```python
from build123d import *

# Parameters (mm, degrees)
F0_W           = 6
F0_H           = 3
F1_DEPTH       = 16
F3_D           = 2
F3_DEPTH       = 5
F3_CBORE_D     = 4
F3_CBORE_DEPTH = 1
F3_TIP         = 0.600860619
F5_D           = 2
F5_DEPTH       = 5
F5_CBORE_D     = 4
F5_CBORE_DEPTH = 1
F5_TIP         = 0.600860619
F6_SIZE        = 4
F8_D           = 3
F8_CBORE_D     = 6
F8_CBORE_DEPTH = 1
F9_SIZE        = 1
F10_SIZE       = 2


with BuildPart() as f1:
    # F0 (on Front) → F1 (new body, symmetric)
    with BuildSketch(Plane.XZ):
        with Locations((-6, 17.5)):
            Rectangle(F0_W, F0_H)
        Polygon((0, -19), (0, 19), (-3, 19), (-3, 16), (-3, -16), (-3, -19), align=None)
        with Locations((-6, -17.5)):
            Rectangle(F0_W, F0_H)
    extrude(amount=F1_DEPTH, both=True)

    # F3
    with Locations(Plane.XY.offset(19)):
        with Locations((-5.5, 8), (-5.5, -8)):
            CounterBoreHole(F3_D / 2, F3_CBORE_D / 2, F3_CBORE_DEPTH, depth=F3_DEPTH)
            with Locations((0, 0, -(F3_DEPTH + F3_TIP / 2))):  # 118° drill point
                Cone(0, F3_D / 2, F3_TIP, mode=Mode.SUBTRACT)

    # F5
    with Locations(Plane(origin=(0, 0, -19), x_dir=(1, 0, 0), z_dir=(0, 0, -1))):
        with Locations((-5.5, -8), (-5.5, 8)):
            CounterBoreHole(F5_D / 2, F5_CBORE_D / 2, F5_CBORE_DEPTH, depth=F5_DEPTH)
            with Locations((0, 0, -(F5_DEPTH + F5_TIP / 2))):  # 118° drill point
                Cone(0, F5_D / 2, F5_TIP, mode=Mode.SUBTRACT)

    # F6
    f6_edges = [f1.edges().sort_by_distance(p)[0] for p in [
        (-9, -16, 17.5),
        (-9, 16, 17.5),
        (-9, 16, -17.5),
        (-9, -16, -17.5),
    ]]
    chamfer(f6_edges, length=F6_SIZE)

    # F8 (through all)
    with Locations(Plane(origin=(-3, 0, 0), x_dir=(0, -1, 0), z_dir=(-1, 0, 0))):
        with Locations((0, 8), (0, -8)):
            CounterBoreHole(F8_D / 2, F8_CBORE_D / 2, F8_CBORE_DEPTH)

    # F9
    f9_edges = [f1.edges().sort_by_distance(p)[0] for p in [
        (-2.5, 16, 19),
        (-7, 14, 19),
        (-9, 0, 19),
        (-7, -14, 19),
        (-2.5, -16, 19),
        (-2.5, 16, -19),
        (-7, 14, -19),
        (-9, 0, -19),
        (-7, -14, -19),
        (-2.5, -16, -19),
    ]]
    chamfer(f9_edges, length=F9_SIZE)

    # F10
    f10_edges = [f1.edges().sort_by_distance(p)[0] for p in [
        (0, 16, 0),
        (0, -16, 0),
    ]]
    chamfer(f10_edges, length=F10_SIZE)


solid = f1.part
```
The model under review builds one solid part; all positions refer to its coordinate system, in mm. A direction names the side the tool comes from. Give positions to 0.01 mm unless a question says otherwise; leave off trailing zeros. Write each loop counter-clockwise with the first axis right and the second up, starting at its lowest first coordinate (ties: lowest second). Pieces come first, ordered by that corner, then holes. Notation, with made-up numbers: (4.25, 27) - (46.25, 27) arc R35 cw to (46.25, 66) - close; hole circle Ø6 at (42, 22). An arc over 180 degrees is marked (long way). Answer in a Markdown table with one row per item. Add a question column.
1. We need section C-C on y = -4.5. Write out the cut boundary in (x, z).
2. We need section A-A on z = -8. Write out the cut boundary in (x, y), then the cut area to 3 significant figures.
3. Insertion check: P1, Ø3, axis at x = -5.5, y = 8, coming from the +Z side; P2, Ø1.5, axis at y = 12.5, z = 8.5, coming from the -X side; P3, Ø1.2, axis at x = -5, y = -8.5, coming from the -Z side; P4, Ø1.6, axis at x = -5.5, y = 8, coming from the -Z side. Each pin has a flat end and moves straight along its axis. Give the tip position at first contact, or say it passes through.
4. We need section D-D on z = -14. Write out the cut boundary in (x, y).
5. Tool access review of faces 5 (the flat face through (-4.6, 7.1, 18)), 6 (the flat face through (-3, -15.5, -18.5)), 7 (the flat face through (-7, -14, 17)), 8 (the flat face through (-6, 0, 16)), 9 (the flat face through (-4.6, -7.1, -18)): name each direction out of +Z, -Z, +X, -X, +Y, -Y from which nothing blocks a thin tool from reaching the whole face with its end or side.
6. We need section B-B on y = 8. Write out the cut boundary in (x, z), then the cut area to 3 significant figures.
7. Draft analysis for pull direction X (two halves, no side actions). For faces 1 (the flat face through (0, 0, 0)), 2 (the flat face through (-3, 15.5, 18.5)), 3 (the cylindrical face through (-5.37, 8.99, 16.99)), 4 (the cylindrical face through (-5.37, 7.01, -16.99)), state which applies: +X half, -X half, draft (parallel to the pull), parting line (faces both ways), or undercut.
8. Wall thickness on line 1 along Z through (x, y) = (-2.6, 0); line 2 along Z through (x, y) = (-5.5, 5.5); line 3 along Z through (x, y) = (-0.45, 0): over which ranges is each line inside the solid? List them lowest first. Write a range as [from, to].
Ans:
| question | item | result |
|---|---|---|
| 1 | outline | (-9, -18) - (-8, -19) - (0, -19) - (0, 19) - (-8, 19) - (-9, 18) - (-9, 16) - (-3, 16) - (-3, -16) - (-9, -16) - close |
| 2 | outline | (-3, -16) - (-2, -16) - (0, -14) - (0, -1.5) - (-2, -1.5) - (-2, -3) - (-3, -3) - close; (-3, 3) - (-2, 3) - (-2, 1.5) - (0, 1.5) - (0, 14) - (-2, 16) - (-3, 16) - close |
| 2 | area | 80.0 mm^2 |
| 3 | P1 | stops at z = 18 |
| 3 | P2 | stops at x = -3 |
| 3 | P3 | stops at z = -18 |
| 3 | P4 | passes through |
| 4 | outline | (-3, -16) - (-2, -16) - (0, -14) - (0, 14) - (-2, 16) - (-3, 16) - close |
| 5 | face 5 | +Z |
| 5 | face 6 | -Z, +X, -X, -Y |
| 5 | face 7 | +Z, -Z, -X, -Y |
| 5 | face 8 | -X, +Y, -Y |
| 5 | face 9 | -Z |
| 6 | outline | (-9, -18) - (-8, -19) - (-7.5, -19) - (-7.5, -18) - (-6.5, -18) - (-6.5, -16) - (-9, -16) - close; (-9, 16) - (-6.5, 16) - (-6.5, 18) - (-7.5, 18) - (-7.5, 19) - (-8, 19) - (-9, 18) - close; (-4.5, -18) - (-3.5, -18) - (-3.5, -19) - (0, -19) - (0, 19) - (-3.5, 19) - (-3.5, 18) - (-4.5, 18) - (-4.5, 16) - (-3, 16) - (-3, -16) - (-4.5, -16) - close |
| 6 | area | 133 mm^2 |
| 7 | face 1 | +X half |
| 7 | face 2 | draft |
| 7 | face 3 | undercut |
| 7 | face 4 | undercut |
| 8 | line 1 | z = [-19, -11], [-5, 5], [11, 19] |
| 8 | line 2 | z = [-19, -16], [16, 19] |
| 8 | line 3 | z = [-19, -9.5], [-6.5, 6.5], [9.5, 19] |
